Work out the finished part from the listing and answer in its coordinate system (mm). Face numbers are marked on the shaded views. A direction names the side the tool comes from. Round coordinates to 2 decimals unless told otherwise and drop trailing zeros. Order: outer loops, then holes, each group sorted by start corner. A loop starts at its lowest first (then second) coordinate and runs counter-clockwise, first axis right, second up. Notation, with made-up numbers: M -6,46.5 L 0,46.5 A32 cw 0,82.5 Z; hole C 74,78 d7. An arc over 180 degrees is marked long. Answer as a JSON object with one key per item and string values. Group by question number.
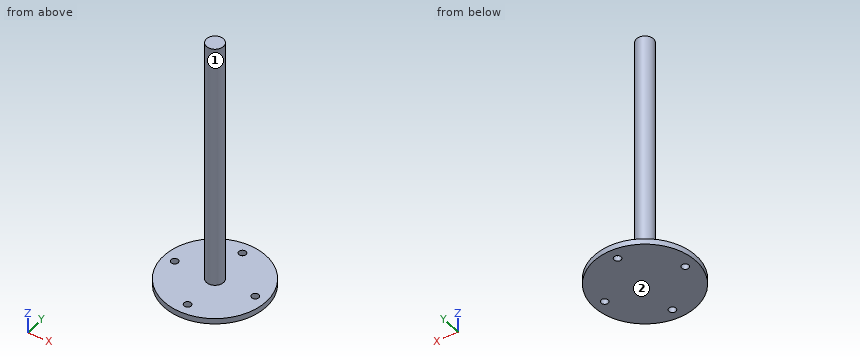
from build123d import *

# Parameters (mm, degrees)
SKETCH1_R           = 57.15
SKETCH1_R_2         = 3.96875
BOSS_EXTRUDE1_DEPTH = 6.35
SKETCH2_R           = 9.525
BOSS_EXTRUDE2_DEPTH = 279.4


with BuildPart() as part:
    # Sketch1 → Boss-Extrude1 (new body)
    with BuildSketch(Plane.XY):
        Circle(SKETCH1_R)
        with Locations((0, 44.45)):
            Circle(SKETCH1_R_2, mode=Mode.SUBTRACT)
        with Locations((44.45, 0)):
            Circle(SKETCH1_R_2, mode=Mode.SUBTRACT)
        with Locations((0, -44.45)):
            Circle(SKETCH1_R_2, mode=Mode.SUBTRACT)
        with Locations((-44.45, 0)):
            Circle(SKETCH1_R_2, mode=Mode.SUBTRACT)
    extrude(amount=BOSS_EXTRUDE1_DEPTH)

    # Sketch2 → Boss-Extrude2 (add)
    with BuildSketch(Plane.XY.offset(6.35)):
        Circle(SKETCH2_R)
    extrude(amount=BOSS_EXTRUDE2_DEPTH)


solid = part.part
Item 1: Find section A-A (x = 0). Give the vertices of the cut face in (y, z) (3 decimals), and give its area (3 significant figures).
Item 2: Find section C-C (z = 79.5). Give the vertices of the cut face in (x, y) (3 decimals).
Item 3: Consider L1, parallel to Y at x = 0, z = 4.75; L2, parallel to Z at x = 39, y = 38; L3, parallel to Y at x = -44.45, z = 2. Determine where each line is inside the solid, lowest interval first.
Item 4: Each of these flat-tipped pins is pushed along its axis until it touches: pin 1 (3 mm diameter, centred on x = -13, y = 15.5, fed in from -Z); pin 2 (9 mm diameter, centred on x = 44.45, y = 0, fed in from +Z); pin 3 (10 mm diameter, centred on y = -18.5, z = 240.5, fed in from +X). Where does it stop, or does it pass through?
Item 5: Find section B-B (y = 44.45). Give the vertices of the cut face in (x, z), and give its area (3 significant figures).
Item 6: A tool of negligible diameter and unlimited length cuts with its end or side. For the marked faces 1 and 2, from which of +Z, -Z, +X, -X, +Y, -Y can it reach the whole face along a straight path? Write none if from no direction.
Responses:
{
 "1": {"outline": "M -57.15,0 L -48.419,0 L -48.419,6.35 L -57.15,6.35 Z; M -40.481,0 L 40.481,0 L 40.481,6.35 L 9.525,6.35 L 9.525,285.75 L -9.525,285.75 L -9.525,6.35 L -40.481,6.35 Z; M 48.419,0 L 57.15,0 L 57.15,6.35 L 48.419,6.35 Z", "area": "5,950 mm^2"},
 "2": {"outline": "C 0,0 d19.05"},
 "3": {"L1": "y = -57.15 to -48.42, -40.48 to 40.48, 48.42 to 57.15", "L2": "z = 0 to 6.35", "L3": "y = -35.92 to -3.97, 3.97 to 35.92"},
 "4": {"pin 1": "stops at z = 0", "pin 2": "stops at z = 6.35", "pin 3": "passes through"},
 "5": {"outline": "M -35.92,0 L -3.97,0 L -3.97,6.35 L -35.92,6.35 Z; M 3.97,0 L 35.92,0 L 35.92,6.35 L 3.97,6.35 Z", "area": "406 mm^2"},
 "6": {"face 1": "+Z", "face 2": "-Z, +X, -X, +Y, -Y"}
}
